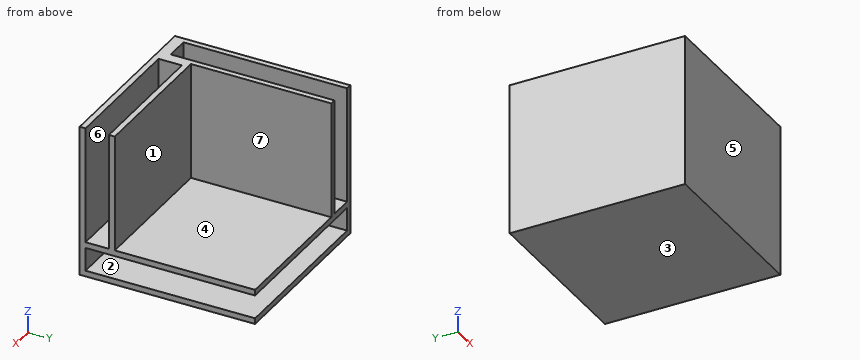
```python
from build123d import *

# Parameters (mm, degrees)
SKETCH1_W            = 30
SKETCH1_H            = 30
BOSS_EXTRUDE1_DEPTH  = 6
BOSS_EXTRUDE4_DEPTH  = 20
SKETCH4_W            = 2
SKETCH4_H            = 2
BOSS_EXTRUDE6_DEPTH  = 20
SKETCH5_W            = 24
SKETCH5_H            = 6
BOSS_EXTRUDE7_DEPTH  = 20
SHELL2_START         = 7
SHELL2_DEPTH         = 23
SHELL2_START_2       = 1
SHELL2_2_DEPTH       = 4
SHELL2_START_3       = 5
SHELL2_3_OUTLINE_W   = 29
SHELL2_3_OUTLINE_H   = 4
SHELL2_3_DEPTH       = 2
SKETCH7_W            = 23
SKETCH7_H            = 1
BOSS_EXTRUDE8_DEPTH  = 5
SKETCH9_W            = 1.075143629
SKETCH9_H            = 23
BOSS_EXTRUDE9_DEPTH  = 5
SKETCH10_W           = 4
SKETCH10_H           = 23
CUT_EXTRUDE1_DEPTH   = 10
SKETCH11_W           = 23
SKETCH11_H           = 4
CUT_EXTRUDE2_DEPTH   = 10
BOSS_EXTRUDE11_DEPTH = 20
SKETCH14_W           = 4
SKETCH14_H           = 19.924856371
CUT_EXTRUDE4_DEPTH   = 5


# Read off the part's stored shape, not the designer's step: Shell2
with BuildPart() as part:
    # Sketch1 → Boss-Extrude1 (new body)
    with BuildSketch(Plane.XY):
        with Locations((15, 15)):
            Rectangle(SKETCH1_W, SKETCH1_H)
    extrude(amount=BOSS_EXTRUDE1_DEPTH)

    # Sketch2 → Boss-Extrude4 (add)
    with BuildSketch(Plane.XY.offset(6)):
        Polygon((5, 6), (6, 6), (6, 30), (0, 30), (0, 6), align=None)
    extrude(amount=BOSS_EXTRUDE4_DEPTH)

    # Sketch4 → Boss-Extrude6 (add)
    with BuildSketch(Plane.XY.offset(6)):
        with Locations((5, 5)):
            Rectangle(SKETCH4_W, SKETCH4_H)
    extrude(amount=BOSS_EXTRUDE6_DEPTH)

    # Sketch5 → Boss-Extrude7 (add)
    with BuildSketch(Plane.XY.offset(6)):
        with Locations((18, 3)):
            Rectangle(SKETCH5_W, SKETCH5_H)
    extrude(amount=BOSS_EXTRUDE7_DEPTH)

    # Shell2 outline → Shell2 (cut)
    with BuildSketch(Plane(origin=(0, 0, 0), x_dir=(1, 0, 0), z_dir=(0, 1, 0)).offset(SHELL2_START)):
        Polygon((5, -5), (30, -5), (30, -1), (1, -1), (1, -25), (5, -25), align=None)
    extrude(amount=SHELL2_DEPTH, mode=Mode.SUBTRACT)

    # Shell2 2 outline → Shell2 2 (cut)
    with BuildSketch(Plane(origin=(0, 0, 0), x_dir=(1, 0, 0), z_dir=(0, 1, 0)).offset(SHELL2_START_2)):
        Polygon((7, -5), (7, -25), (30, -25), (30, -1), (1, -1), (1, -5), align=None)
    extrude(amount=SHELL2_2_DEPTH, mode=Mode.SUBTRACT)

    # Shell2 3 outline → Shell2 3 (cut)
    with BuildSketch(Plane(origin=(0, 0, 0), x_dir=(1, 0, 0), z_dir=(0, 1, 0)).offset(SHELL2_START_3)):
        with Locations((15.5, -3)):
            Rectangle(SHELL2_3_OUTLINE_W, SHELL2_3_OUTLINE_H)
    extrude(amount=SHELL2_3_DEPTH, mode=Mode.SUBTRACT)

    # Sketch7 → Boss-Extrude8 (add)
    with BuildSketch(Plane.XZ.offset(-5)):
        with Locations((18.5, 5.5)):
            Rectangle(SKETCH7_W, SKETCH7_H)
    extrude(amount=BOSS_EXTRUDE8_DEPTH)

    # Sketch9 → Boss-Extrude9 (add)
    with BuildSketch(Plane.ZY.offset(-5)):
        with Locations((5.537571814, 18.5)):
            Rectangle(SKETCH9_W, SKETCH9_H)
    extrude(amount=BOSS_EXTRUDE9_DEPTH)

    # Sketch10 → Cut-Extrude1 (cut)
    with BuildSketch(Plane.XY.offset(26)):
        with Locations((3, 18.5)):
            Rectangle(SKETCH10_W, SKETCH10_H)
    extrude(amount=-CUT_EXTRUDE1_DEPTH, mode=Mode.SUBTRACT)

    # Sketch11 → Cut-Extrude2 (cut)
    with BuildSketch(Plane.XY.offset(26)):
        with Locations((18.5, 3)):
            Rectangle(SKETCH11_W, SKETCH11_H)
    extrude(amount=-CUT_EXTRUDE2_DEPTH, mode=Mode.SUBTRACT)

    # Sketch12 → Boss-Extrude11 (add)
    with BuildSketch(Plane.XY.offset(6)):
        Polygon((6, 0), (6, 4), (4, 4), (4, 6), (0, 6), (0, 0), align=None)
    extrude(amount=BOSS_EXTRUDE11_DEPTH)

    # Sketch14 → Cut-Extrude4 (cut)
    with BuildSketch(Plane(origin=(0, 7, 0), x_dir=(1, 0, 0), z_dir=(0, 1, 0))):
        with Locations((3, -16.037571815)):
            Rectangle(SKETCH14_W, SKETCH14_H)
    extrude(amount=-CUT_EXTRUDE4_DEPTH, mode=Mode.SUBTRACT)


solid = part.part
```
Here's how the part is built. I have some questions about the finished solid (model axes, mm). Face numbers are marked on the shaded views. A direction names the side the tool comes from. Give positions to 0.01 mm unless a question says otherwise; leave off trailing zeros. Order: outer loops, then holes, each group sorted by start corner. A loop starts at its lowest first (then second) coordinate and runs counter-clockwise, first axis right, second up. Notation, with made-up numbers: M 12,-34.75 L 38,-34.75 A14 ccw 38,-12.75 Z; hole C -16.5,53.5 d8. An arc over 180 degrees is marked long. Use a Markdown table: item, result. Add a question column.
1. On a 3-axis mill with a long thin cutter (end or side, diameter ignored), from which of +Z, -Z, +X, -X, +Y, -Y can I reach the whole of each face in a straight line? I mean the marked faces 5, 6 and 7. Say none if no direction works.
2. Suppose I cut it at C-C (x = 2.5). List the corners of the cut face in (y, z) for me, and give its area (3 significant figures).
3. For pin 1 Ø2 at (y, z) = (3.5, 9.5) entering from +X; pin 2 Ø10 at (x, z) = (21, 17.5) entering from +Y; pin 3 Ø1.2 at (x, z) = (2, 13.5) entering from +Y, each with a flat end and sliding along its axis, tell me the tip position at first contact or that it passes through.
4. Suppose I cut it at A-A (y = 24). List the corners of the cut face in (x, z) for me.
5. If we mould it in two halves opening along Z, with no side actions, what happens to the marked faces 1, 2, 3 and 4? For each: +Z half, -Z half, draft (parallel to the pull), parting line (faces both ways), or undercut.
6. Suppose I cut it at D-D (z = 3.5). List the corners of the cut face in (x, y) for me.
7. I need wall thicknesses on probe 1 along Z at (x, y) = (6.25, 17.5). Which ranges of the line are inside material? Lowest first, please. Write a range as from..to.
8. Suppose I cut it at B-B (z = 17.5). List the corners of the cut face in (x, y) for me.
Results list:
| question | item | result |
|---|---|---|
| 1 | face 5 | +Z, -Z, +X, -X, -Y |
| 1 | face 6 | +Z, +X |
| 1 | face 7 | +Z, +X, +Y |
| 2 | outline | M 0,0 L 30,0 L 30,1 L 1,1 L 1,5 L 30,5 L 30,6.08 L 2,6.08 L 2,26 L 0,26 Z |
| 2 | area | 106 mm² |
| 3 | pin 1 | stops at x = 7 |
| 3 | pin 2 | stops at y = 6 |
| 3 | pin 3 | stops at y = 2 |
| 4 | outline | M 0,0 L 30,0 L 30,1 L 1,1 L 1,5 L 30,5 L 30,6 L 6,6 L 6,26 L 5,26 L 5,6.08 L 1,6.08 L 1,26 L 0,26 Z |
| 5 | face 1 | draft |
| 5 | face 2 | undercut |
| 5 | face 3 | -Z half |
| 5 | face 4 | +Z half |
| 6 | outline | M 0,0 L 30,0 L 30,1 L 1,1 L 1,30 L 0,30 Z |
| 7 | probe 1 | z = 0..1, 5..6 |
| 8 | outline | M 0,0 L 30,0 L 30,1 L 7,1 L 7,5 L 30,5 L 30,6 L 6,6 L 6,30 L 5,30 L 5,2 L 1,2 L 1,30 L 0,30 Z |
